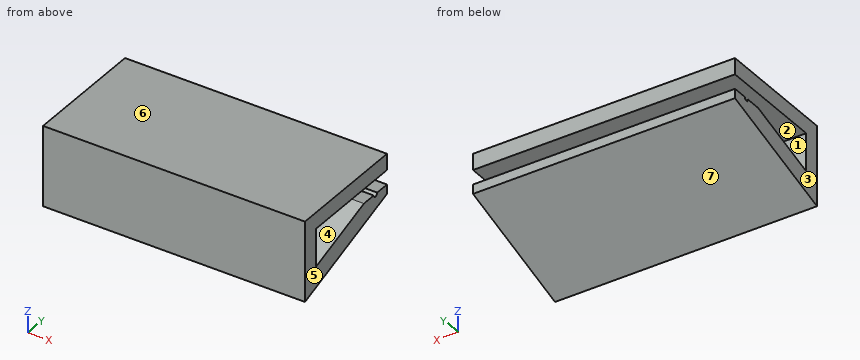
```python
from build123d import *

# Parameters (mm, degrees)
BOSS_EXTRUDE1_DEPTH = 10


with BuildPart() as part:
    # Sketch1 → Boss-Extrude1 (new, symmetric)
    with BuildSketch(Plane(origin=(0, 0, 0), x_dir=(0, 0, -1), z_dir=(1, 0, 0))):
        with BuildLine():
            Line((0, 0), (6.116419195, 0))
            Line((6.116419195, 0), (3.055144814, 9.421633765))
            Line((3.055144814, 9.421633765), (2.339181313, 9.421633765))
            Line((2.339181313, 9.421633765), (2.339181313, 8.296337322))
            ThreePointArc((2.339181313, 8.296337322), (2.539181313, 8.096337322), (2.339181313, 7.896337322))
            Line((2.339181313, 7.896337322), (2.339181313, 6.771040879))
            Line((2.339181313, 6.771040879), (4.136591443, 1.239181313))
            Line((4.136591443, 1.239181313), (1.239181313, 1.239181313))
            Line((1.239181313, 1.239181313), (1.239181313, 9.421633765))
            Line((1.239181313, 9.421633765), (0, 9.421633765))
            Line((0, 9.421633765), (0, 0))
        make_face()
    extrude(amount=BOSS_EXTRUDE1_DEPTH, both=True)


solid = part.part
```
Part model, mm, in its own coordinate system. Face numbers are marked on the shaded views. A direction names the side the tool comes from. Coordinates: 2 decimals unless noted, no trailing zeros. Order: outer loops, then holes, each group sorted by start corner. A loop starts at its lowest first (then second) coordinate and runs counter-clockwise, first axis right, second up. Notation, with made-up numbers: (-20.75, -26) -> (-3.75, -26) arc R29 cw to (-3.75, -1) -> close; hole circle Ø4 at (23.25, -17.5). An arc over 180 degrees is marked (long way). Put each result on its own line as item: value. Start each with the question number.
(1) Band-saw the part on B-B (x = 1.5). Give the cut face in (y, z).
(2) Band-saw the part on D-D (y = 9). Give the cut face in (x, z).
(3) Mould opens along Z. For the marked faces 4, 5, 6 and 7 say: pulls with the +Z half, pulls with the -Z half, needs draft (parallel to the pull), parting line crosses it, or undercut.
(4) Band-saw the part on C-C (z = -1.5). Give the cut face in (x, y), then the cut area to 3 significant figures.
(5) Probe line 1 along Y through (x, z) = (5, -1.75); line 2 along Z through (x, y) = (-6.5, 2.75); line 3 along Z through (x, y) = (-1, 2.25). List the from-to ranges inside material, lowest first. Write a range as [from, to].
(6) Which spindle directions (+Z, -Z, +X, -X, +Y, -Y) get a long thin tool onto all of the face, cutting with end or side? Do the marked faces 1, 2 and 3. Say none if no direction does.
(7) Pin check, flat tips, straight feed: pin 1 Ø2 at (x, y) = (0.5, 5.5) entering from +Z; pin 2 Ø2.5 at (x, y) = (3.5, 5.5) entering from -Z. Stop position of each tip, or through.
(8) Band-saw the part on A-A (y = 7.25). Give the cut face in (x, z), then the cut area to 3 significant figures.
Determined:
1. outline: (0, -6.12) -> (9.42, -3.06) -> (9.42, -2.34) -> (8.3, -2.34) arc R0.2 cw to (7.9, -2.34) -> (6.77, -2.34) -> (1.24, -4.14) -> (1.24, -1.24) -> (9.42, -1.24) -> (9.42, 0) -> (0, 0) -> close
2. outline: (-10, -3.19) -> (10, -3.19) -> (10, -2.34) -> (-10, -2.34) -> close; (-10, -1.24) -> (10, -1.24) -> (10, 0) -> (-10, 0) -> close
3. face 4: undercut
3. face 5: needs draft
3. face 6: pulls with the +Z half
3. face 7: pulls with the -Z half
4. outline: (-10, 0) -> (10, 0) -> (10, 1.24) -> (-10, 1.24) -> close
4. area: 24.8 mm²
5. line 1: y = [0, 1.24]
5. line 2: z = [-5.22, -3.65], [-1.24, 0]
5. line 3: z = [-5.39, -3.81], [-1.24, 0]
6. face 1: +X, -X
6. face 2: +X, -X, +Y
6. face 3: +Z, -Z, -X, +Y, -Y
7. pin 1: stops at z = 0
7. pin 2: stops at z = -4.74
8. outline: (-10, -3.76) -> (10, -3.76) -> (10, -2.34) -> (-10, -2.34) -> close; (-10, -1.24) -> (10, -1.24) -> (10, 0) -> (-10, 0) -> close
8. area: 53.2 mm²
